Input: part model. Units: mm. Frame: model coordinates. Coordinates: 2 decimals unless noted, no trailing zeros. Order: outer loops, then holes, each group sorted by start corner. A loop starts at its lowest first (then second) coordinate and runs counter-clockwise, first axis right, second up. Notation, with made-up numbers: (77, 82) - (132, 82) arc R18 cw to (132, 93) - close; hole circle Ø11 at (73.25, 23.25). An arc over 180 degrees is marked (long way). Use a Markdown table: item, result. Add a question column.
from build123d import *

# Parameters (mm, degrees)
SKETCH1_W           = 150
SKETCH1_H           = 150
BOSS_EXTRUDE1_DEPTH = 12.7
SKETCH2_W           = 10.53028371
SKETCH2_H           = 7.9375
SKETCH2_R           = 2.5
CUT_EXTRUDE1_DEPTH  = 12.7


with BuildPart() as part:
    # Sketch1 → Boss-Extrude1 (new body)
    with BuildSketch(Plane(origin=(0, 0, 0), x_dir=(1, 0, 0), z_dir=(0, 1, 0))):
        with Locations((75, 75)):
            Rectangle(SKETCH1_W, SKETCH1_H)
    extrude(amount=BOSS_EXTRUDE1_DEPTH)

    # Sketch2 → Cut-Extrude1 (cut)
    with BuildSketch(Plane(origin=(0, 12.7, 0), x_dir=(1, 0, 0), z_dir=(0, 1, 0))):
        with BuildLine():
            ThreePointArc((80.265141855, 67.0625), (83.392737967, 70.495827), (84.525, 75))
            Line((84.525, 75), (80.265141855, 75))
            Line((80.265141855, 75), (80.265141855, 67.0625))
        make_face()
        with BuildLine():
            Line((80.265141855, 75), (84.525, 75))
            ThreePointArc((84.525, 75), (83.392737967, 79.504173), (80.265141855, 82.9375))
            Line((80.265141855, 82.9375), (80.265141855, 75))
        make_face()
        with BuildLine():
            Line((69.734858145, 67.0625), (69.734858145, 75))
            Line((69.734858145, 75), (65.475, 75))
            ThreePointArc((65.475, 75), (66.607262033, 70.495827), (69.734858145, 67.0625))
        make_face()
        with BuildLine():
            Line((65.475, 75), (69.734858145, 75))
            Line((69.734858145, 75), (69.734858145, 82.9375))
            ThreePointArc((69.734858145, 82.9375), (66.607262033, 79.504173), (65.475, 75))
        make_face()
        with Locations((75, 78.96875)):
            Rectangle(SKETCH2_W, SKETCH2_H)
        with Locations((75, 71.03125)):
            Rectangle(SKETCH2_W, SKETCH2_H)
        with Locations((10, 140)):
            Circle(SKETCH2_R)
        with Locations((140, 140)):
            Circle(SKETCH2_R)
        with Locations((140, 10)):
            Circle(SKETCH2_R)
        with Locations((10, 10)):
            Circle(SKETCH2_R)
    extrude(amount=-CUT_EXTRUDE1_DEPTH, mode=Mode.SUBTRACT)


solid = part.part
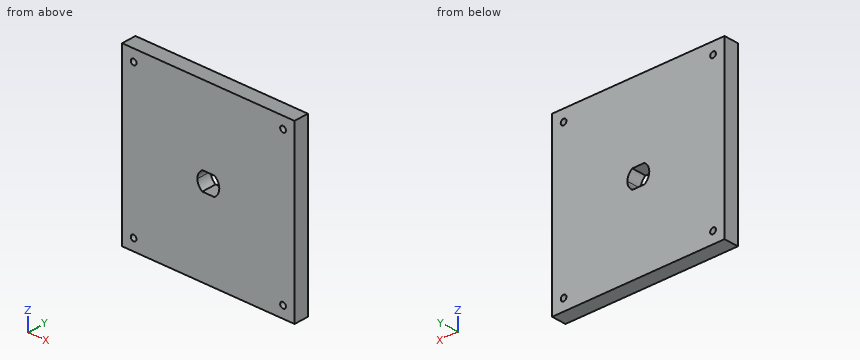
1) Cut plane C-C (z = -78.5). Return the cut outline in (x, y).
2) Cut plane D-D (z = -10). Return the cut outline in (x, y), and give its area (3 significant figures).
3) Cut plane B-B (x = 76.5). Return the cut outline in (y, z), and give its area (3 significant figures).
4) Material intervals for L1, parallel to X at y = 7.5, z = -10; L2, parallel to Z at x = 140, y = 4.5; L3, parallel to Z at x = 9.5, y = 11.5, sorted ascending.
5) Cut plane A-A (y = 7.25). State how many separate pieces and enclosed holes the cut face has, and give its area (3 significant figures).
Computed:
| question | item | result |
|---|---|---|
| 1 | outline | (0, 0) - (66.14, 0) - (66.14, 12.7) - (0, 12.7) - close; (83.86, 0) - (150, 0) - (150, 12.7) - (83.86, 12.7) - close |
| 2 | outline | (0, 0) - (7.5, 0) - (7.5, 12.7) - (0, 12.7) - close; (12.5, 0) - (137.5, 0) - (137.5, 12.7) - (12.5, 12.7) - close; (142.5, 0) - (150, 0) - (150, 12.7) - (142.5, 12.7) - close |
| 2 | area | 1,780 mm2 |
| 3 | outline | (0, -150) - (12.7, -150) - (12.7, -82.94) - (0, -82.94) - close; (0, -67.06) - (12.7, -67.06) - (12.7, 0) - (0, 0) - close |
| 3 | area | 1,700 mm2 |
| 4 | L1 | x = 0 to 7.5, 12.5 to 137.5, 142.5 to 150 |
| 4 | L2 | z = -150 to -142.5, -137.5 to -12.5, -7.5 to 0 |
| 4 | L3 | z = -150 to -142.45, -137.55 to -12.45, -7.55 to 0 |
| 5 | separate pieces | 1 |
| 5 | enclosed holes | 5 |
| 5 | area | 22,200 mm2 |
